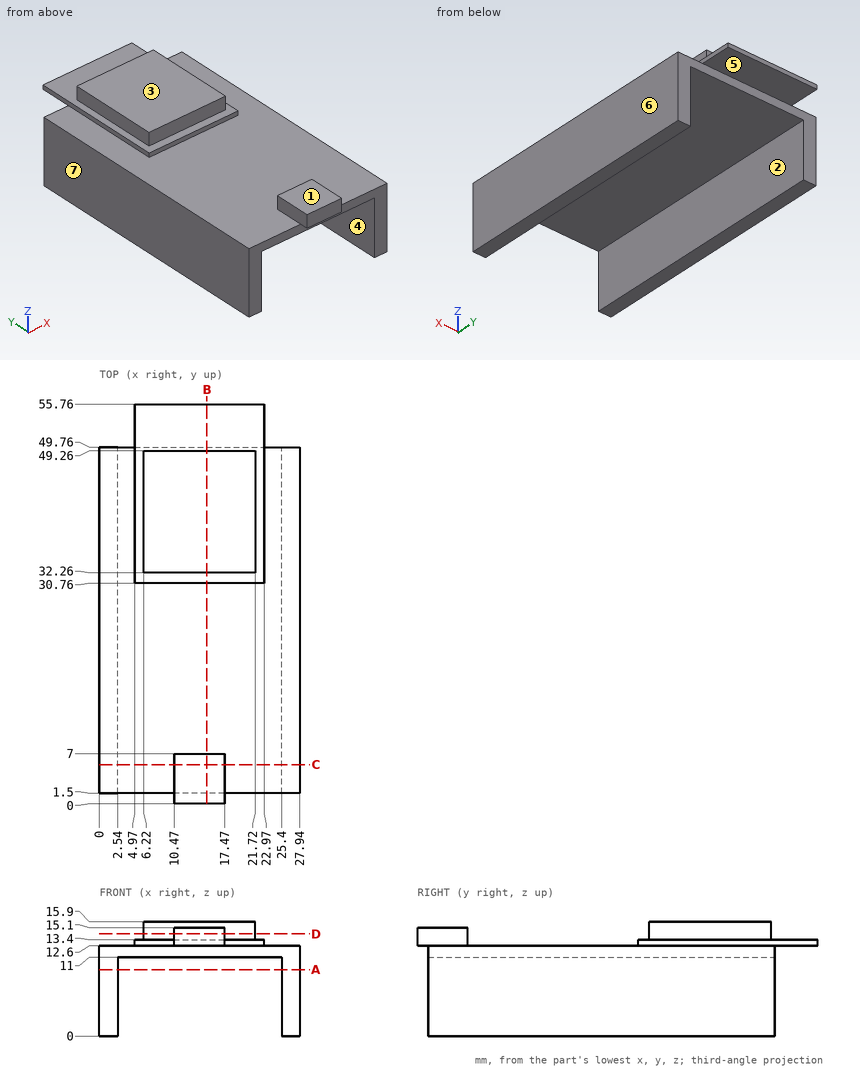
Source: three-view drawing plus pictorial views. Frame: mm from the lowest corner of the part. A direction names the side the tool comes from. Round coordinates to 2 decimals unless told otherwise and drop trailing zeros. Order: outer loops, then holes, each group sorted by start corner. A loop starts at its lowest first (then second) coordinate and runs counter-clockwise, first axis right, second up. Notation, with made-up numbers: (69.25, 58) -> (74.25, 58) arc R22 cw to (74.25, 87) -> close; hole circle Ø8 at (-2, 79.25). An arc over 180 degrees is marked (long way). Use one line per item in the form item = value. Start each with the question number.
1. Cut plane C-C (y = 5.5). Return the cut outline in (x, z), then the cut area to 3 significant figures.
2. Cut plane A-A (z = 9.25). Return the cut outline in (x, y), then the cut area to 3 significant figures.
3. Draft query along X for the marked faces 4, 5, 6 and 7. Return one class per face: pulls with the +X half, pulls with the -X half, needs draft (parallel to the pull), parting line crosses it, or undercut.
4. Cut plane B-B (x = 15). Return the cut outline in (y, z).
5. Cut plane D-D (z = 14.25). Return the cut outline in (x, y), then the cut area to 4 significant figures.
6. Reachability of the marked faces 1, 2 and 3 from +Z, -Z, +X, -X, +Y, -Y: full face, straight path, thin tool, end or side. Return the list, or none.
7. Line query: probe 1 along X at (y, z) = (4.5, 3.5); probe 2 along Z at (x, y) = (14.25, 30); probe 3 along Y at (x, z) = (14.5, 13.25). Output: solid intervals per line, ascending.
8. Pin query (flat end, axial travel): pin 1 Ø1 at (x, y) = (22.5, 27) entering from +Z; pin 2 Ø0.8 at (y, z) = (41.5, 15) entering from -X; pin 3 Ø0.6 at (y, z) = (43, 13) entering from +X; pin 4 Ø8 at (x, z) = (15.5, 5.5) entering from -Y. Return the tip coordinate at first contact, or that it passes through.
Solution:
q1.outline = (0, 0) -> (2.54, 0) -> (2.54, 11) -> (25.4, 11) -> (25.4, 0) -> (27.94, 0) -> (27.94, 12.6) -> (17.47, 12.6) -> (17.47, 15.1) -> (10.47, 15.1) -> (10.47, 12.6) -> (0, 12.6) -> close
q1.area = 118 mm^2
q2.outline = (0, 1.5) -> (2.54, 1.5) -> (2.54, 49.76) -> (0, 49.76) -> close; (25.4, 1.5) -> (27.94, 1.5) -> (27.94, 49.76) -> (25.4, 49.76) -> close
q2.area = 245 mm^2
q3.face_4 = undercut
q3.face_5 = needs draft
q3.face_6 = pulls with the +X half
q3.face_7 = pulls with the -X half
q4.outline = (0, 12.6) -> (1.5, 12.6) -> (1.5, 11) -> (49.76, 11) -> (49.76, 12.6) -> (55.76, 12.6) -> (55.76, 13.4) -> (49.26, 13.4) -> (49.26, 15.9) -> (32.26, 15.9) -> (32.26, 13.4) -> (30.76, 13.4) -> (30.76, 12.6) -> (7, 12.6) -> (7, 15.1) -> (0, 15.1) -> close
q5.outline = (6.22, 32.26) -> (21.72, 32.26) -> (21.72, 49.26) -> (6.22, 49.26) -> close; (10.47, 0) -> (17.47, 0) -> (17.47, 7) -> (10.47, 7) -> close
q5.area = 312.5 mm^2
q6.face_1 = +Z, +X, -X, -Y
q6.face_2 = -Z, +Y, -Y
q6.face_3 = +Z, +X, -X, +Y, -Y
q7.probe_1 = 0 to 2.54, 25.4 to 27.94
q7.probe_2 = 11 to 12.6
q7.probe_3 = 0 to 7, 30.76 to 55.76
q8.pin_1 = 12.6
q8.pin_2 = 6.22
q8.pin_3 = 22.97
q8.pin_4 = through
